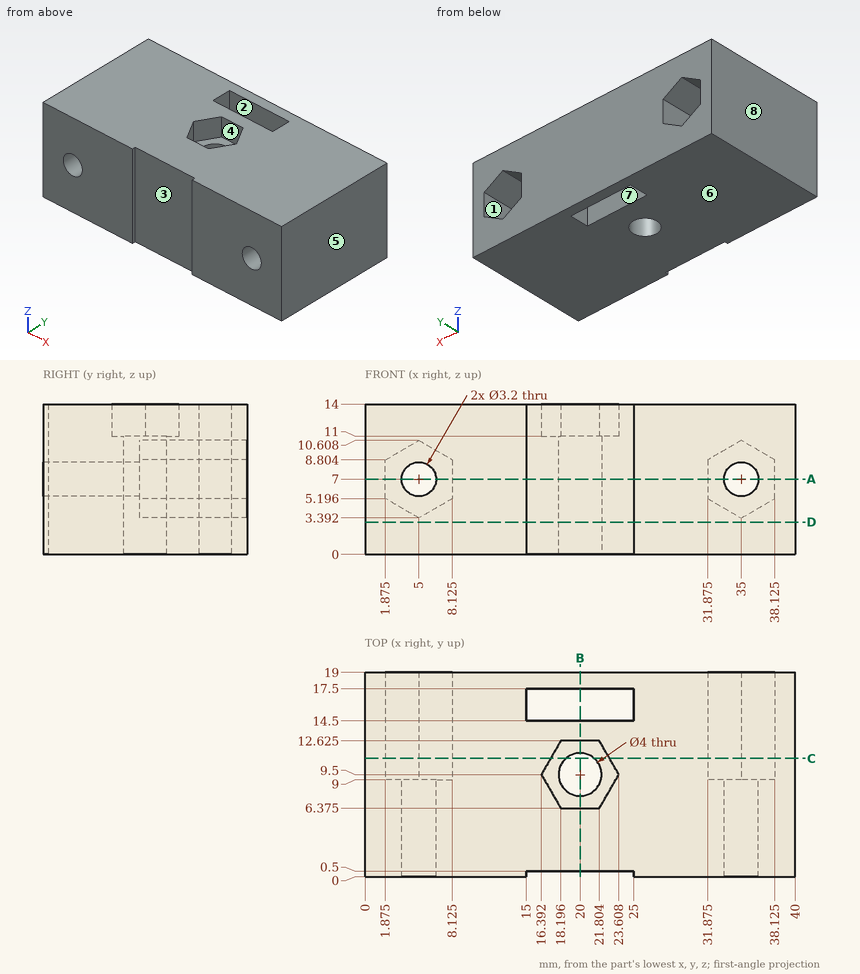
For this review, use the dimensioned drawing (mm, ordinates from the lowest corner) and the shaded views. A direction names the side the tool comes from. Give positions to 0.01 mm unless a question says otherwise; leave off trailing zeros. Order: outer loops, then holes, each group sorted by start corner. A loop starts at its lowest first (then second) coordinate and runs counter-clockwise, first axis right, second up. Notation, with made-up numbers: (17, 67) - (40, 67) arc R17 cw to (40, 91) - close; hole circle Ø2 at (19, 16.5). An arc over 180 degrees is marked (long way). Use a Markdown table: item, result. Add a question column.
(1) Clearance check with flat-ended pins moving along their axes: P1, Ø6, axis at x = 22.5, y = 6, coming from the -Z side; P2, Ø1.5, axis at x = 20.5, z = 12.5, coming from the -Y side; P3, Ø5, axis at x = 5, z = 7, coming from the +Y side; P4, Ø1.9, axis at x = 18.5, y = 10.5, coming from the +Z side. State where each tip first meets the part, or that it passes through.
(2) Mouldability with a two-part tool opening along X and no side actions: class the marked faces 6, 7 and 8 as +X half, -X half, draft (parallel to the pull), parting line (faces both ways), or undercut.
(3) Machinability: for the marked faces 1, 2, 3, 4 and 5, which of the approach directions +Z, -Z, +X, -X, +Y, -Y give a long, thin tool a straight path to every point of the face, cutting with its end or side? Answer none if there is none.
(4) Add section D-D on z = 3. Give the boundary of the cut face in (x, y).
(5) Add section A-A on z = 7. Give the number of separate pieces and of enclosed holes in the cut face, then the cut area to 3 significant figures.
(6) Add section B-B on x = 20. Give the boundary of the cut face in (y, z) (1 decimal), then the cut area to 3 significant figures.
(7) Wall thickness on probe 1 along Y at (x, z) = (20, 6.75); probe 2 along X at (y, z) = (4.5, 7); probe 3 along X at (y, z) = (9.25, 7.75) (1 decimal): over which ranges is each line inside the solid? List them lowest first. Write a range as [from, to].
(8) Add section C-C on y = 11. Give the boundary of the cut face in (x, z) (1 decimal), then the cut area to 3 significant figures.
Report:
| question | item | result |
|---|---|---|
| 1 | P1 | stops at z = 0 |
| 1 | P2 | stops at y = 0.5 |
| 1 | P3 | stops at y = 9 |
| 1 | P4 | stops at z = 11 |
| 2 | face 6 | draft |
| 2 | face 7 | undercut |
| 2 | face 8 | -X half |
| 3 | face 1 | +Y |
| 3 | face 2 | +Z, -Z |
| 3 | face 3 | +Z, -Z, -Y |
| 3 | face 4 | +Z |
| 3 | face 5 | +Z, -Z, +X, +Y, -Y |
| 4 | outline | (0, 0) - (15, 0) - (15, 0.5) - (25, 0.5) - (25, 0) - (40, 0) - (40, 19) - (0, 19) - close; hole (15, 14.5) - (25, 14.5) - (25, 17.5) - (15, 17.5) - close; hole circle Ø4 at (20, 9.5) |
| 5 | separate pieces | 3 |
| 5 | enclosed holes | 2 |
| 5 | area | 530 mm² |
| 6 | outline | (0.5, 0) - (7.5, 0) - (7.5, 11) - (6.4, 11) - (6.4, 14) - (0.5, 14) - close; (11.5, 0) - (14.5, 0) - (14.5, 14) - (12.6, 14) - (12.6, 11) - (11.5, 11) - close; (17.5, 0) - (19, 0) - (19, 14) - (17.5, 14) - close |
| 6 | area | 154 mm² |
| 7 | probe 1 | y = [0.5, 7.5], [11.5, 14.5], [17.5, 19] |
| 7 | probe 2 | x = [0, 3.4], [6.6, 33.4], [36.6, 40] |
| 7 | probe 3 | x = [0, 1.9], [8.1, 18], [22, 31.9], [38.1, 40] |
| 8 | outline | (0, 0) - (18.7, 0) - (18.7, 11) - (17.3, 11) - (17.3, 14) - (0, 14) - close; (21.3, 0) - (40, 0) - (40, 14) - (22.7, 14) - (22.7, 11) - (21.3, 11) - close; hole (1.9, 5.2) - (5, 3.4) - (8.1, 5.2) - (8.1, 8.8) - (5, 10.6) - (1.9, 8.8) - close; hole (31.9, 5.2) - (35, 3.4) - (38.1, 5.2) - (38.1, 8.8) - (35, 10.6) - (31.9, 8.8) - close |
| 8 | area | 447 mm² |
